Design review of the part built by this model. Coordinates are the model's own, in mm. Face numbers are marked on the shaded views. Round coordinates to 2 decimals unless told otherwise and drop trailing zeros. Loops run counter-clockwise (first coordinate to the right, second up) from the corner with the lowest first, then second, coordinate; pieces in that order, holes last. Notation, with made-up numbers: (3.5, -34.75) - (47.5, -34.75) arc R12 ccw to (47.5, -19.75) - close; hole circle Ø4 at (72.5, -9.75). An arc over 180 degrees is marked (long way). Return JSON: item names as keys, results as strings. Group by question number.
(1) The part is to be moulded in two halves that separate along Y. For the marked faces 1, 2 and 3, say which applies: pulls with the +Y half, pulls with the -Y half, needs draft (parallel to the pull), parting line crosses it, or undercut.
(2) Clearance check with flat-ended pins moving along their axes: pin 1 (6 mm diameter, centred on y = -10.5, z = 9.5, fed in from +X); pin 2 (8 mm diameter, centred on y = -8, z = 13.5, fed in from -X); pin 3 (1.5 mm diameter, centred on y = 11.5, z = 5.5, fed in from +X). State where each tip first meets the part, or that it passes through.
(3) Wall thickness on L1, parallel to Y at x = 0, z = 9.75; L2, parallel to Y at x = 0, z = 6.75; L3, parallel to Z at x = 6.5, y = -11: over which ranges is each line inside the solid? List them lowest first. Write a range as [from, to].
(4) We need section A-A, the plane y = 0. Write out the cut boundary in (x, z).
(5) We need section C-C, the plane z = 11.75. Write out the cut boundary in (x, y).
from build123d import *

# Parameters (mm, degrees)
SKETCH_1_R          = 22.5
EXTRUDE_1_DEPTH     = 8
SKETCH_2_R          = 2
SKETCH_3_R          = 10
EXTRUDE_2_DEPTH     = 8
SKETCH_4_R          = 3
CUT_EXTRUDE_1_DEPTH = 36.616007637


with BuildPart() as part:
    # 草图1 → 凸台-拉伸1 (new body)
    with BuildSketch(Plane.XY):
        Circle(SKETCH_1_R)
    extrude(amount=EXTRUDE_1_DEPTH)

    # 草图2 → 切除-旋转1 (revolve, cut)
    with BuildSketch(Plane(origin=(0, 0, 0), x_dir=(1, 0, 0), z_dir=(0, 1, 0)), mode=Mode.PRIVATE) as cut_revolve_1_sk:
        with Locations((-22.5, -4)):
            Circle(SKETCH_2_R)
    revolve(cut_revolve_1_sk.sketch.rotate(Axis((0, 0, 8), (0, 0, -1)), 180), axis=Axis((0, 0, 8), (0, 0, -1)), mode=Mode.SUBTRACT)

    # 草图3 → 凸台-拉伸2 (add)
    with BuildSketch(Plane.XY.offset(8)):
        Circle(SKETCH_3_R)
    extrude(amount=EXTRUDE_2_DEPTH)

    # 草图4 → 切除-拉伸1 (cut, through all)
    with BuildSketch(Plane.XY.offset(16)):
        Circle(SKETCH_4_R)
    extrude(amount=-CUT_EXTRUDE_1_DEPTH, mode=Mode.SUBTRACT)


solid = part.part
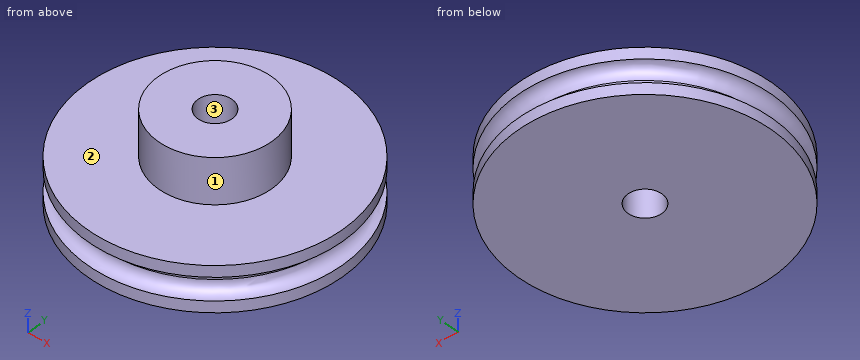
Solutions:
{
 "1": {"face 1": "parting line crosses it", "face 2": "needs draft", "face 3": "undercut"},
 "2": {"pin 1": "x = 21.07", "pin 2": "x = -9.17", "pin 3": "x = 19.66"},
 "3": {"L1": "[-10, -3], [3, 10]", "L2": "[-22.5, -3], [3, 22.5]", "L3": "[0, 8]"},
 "4": {"outline": "(-22.5, 0) - (-3, 0) - (-3, 16) - (-10, 16) - (-10, 8) - (-22.5, 8) - (-22.5, 6) arc R2 cw to (-22.5, 2) - close; (3, 0) - (22.5, 0) - (22.5, 2) arc R2 cw to (22.5, 6) - (22.5, 8) - (10, 8) - (10, 16) - (3, 16) - close"},
 "5": {"outline": "circle Ø20 at (0, 0); hole circle Ø6 at (0, 0)"}
}
